from build123d import *

# Parameters (mm, degrees)
SKETCH4_W           = 30
SKETCH4_H           = 17.5
SKETCH4_R           = 2
BOSS_EXTRUDE2_DEPTH = 5
SKETCH5_W           = 30
SKETCH5_H           = 5
BOSS_EXTRUDE3_DEPTH = 15


with BuildPart() as part:
    # Sketch4 → Boss-Extrude2 (new body)
    with BuildSketch(Plane.XY):
        with Locations((0, 1.25)):
            Rectangle(SKETCH4_W, SKETCH4_H)
        with Locations((10.86, -3.5)):
            Circle(SKETCH4_R, mode=Mode.SUBTRACT)
        with Locations(Location((-10.86, -3.5, 0), (0, 0, 180))):
            Circle(SKETCH4_R, mode=Mode.SUBTRACT)
    extrude(amount=BOSS_EXTRUDE2_DEPTH)

    # Sketch5 → Boss-Extrude3 (add)
    with BuildSketch(Plane.XY):
        with Locations((0, 12.5)):
            Rectangle(SKETCH5_W, SKETCH5_H)
    extrude(amount=BOSS_EXTRUDE3_DEPTH)


solid = part.part
For this review, take the finished solid that the model builds, in its own axes (mm). A direction names the side the tool comes from. Give positions to 0.01 mm unless a question says otherwise; leave off trailing zeros. Order: outer loops, then holes, each group sorted by start corner. A loop starts at its lowest first (then second) coordinate and runs counter-clockwise, first axis right, second up. Notation, with made-up numbers: M 1,-17.5 L 55,-17.5 A13 cw 55,0.5 Z; hole C -0.5,59.5 d7. An arc over 180 degrees is marked long. Answer in a Markdown table with one row per item. Add a question column.
(1) Consider section C-C on z = 3.5. State the section outline as (x, y) points, and give its area (3 significant figures).
(2) Consider section A-A on y = -3.5. State the section outline as (x, z) points.
(3) Consider section B-B on x = 10.75. State the section outline as (y, z) points.
(4) Wall thickness on probe 1 along Y at (x, z) = (10.86, 3.7); probe 2 along Y at (x, z) = (13, 6.75); probe 3 along Z at (x, y) = (5.25, -5.5): over which ranges is each line inside the solid? List them lowest first. Write a range as [from, to].
(5) For faces 1 (the face through (0, 1, 5)), 2 (the face through (-8.862, -3.588, 2.465)), list the 3-axis set-ups (+Z, -Z, +X, -X, +Y, -Y) from which the entire face can be reached by the end or side of a thin tool; tool diameter is ignored.
(6) For pin 1 (9 mm diameter, centred on x = 7.5, y = 4, fed in from +Z), flat-tipped, find the tip position at first contact; note if it passes through.
(7) Mouldability with a two-part tool opening along X and no side actions: class faces 3 (the face through (8.862, -3.412, 2.465)), 4 (the face through (-15, 6, 4)), 5 (the face through (0, 10, 10)), 6 (the face through (15, 6, 4)) as +X half, -X half, draft (parallel to the pull), parting line (faces both ways), or undercut.
(8) Consider section D-D on x = 2.5. State the section outline as (y, z) points.
Evaluation:
| question | item | result |
|---|---|---|
| 1 | outline | M -15,-7.5 L 15,-7.5 L 15,15 L -15,15 Z; hole C -10.86,-3.5 d4; hole C 10.86,-3.5 d4 |
| 1 | area | 650 mm^2 |
| 2 | outline | M -15,0 L -12.86,0 L -12.86,5 L -15,5 Z; M -8.86,0 L 8.86,0 L 8.86,5 L -8.86,5 Z; M 12.86,0 L 15,0 L 15,5 L 12.86,5 Z |
| 3 | outline | M -7.5,0 L -5.5,0 L -5.5,5 L -7.5,5 Z; M -1.5,0 L 15,0 L 15,15 L 10,15 L 10,5 L -1.5,5 Z |
| 4 | probe 1 | y = [-7.5, -5.5], [-1.5, 15] |
| 4 | probe 2 | y = [10, 15] |
| 4 | probe 3 | z = [0, 5] |
| 5 | face 1 | +Z, +X, -X, -Y |
| 5 | face 2 | +Z, -Z |
| 6 | pin 1 | stops at z = 5 |
| 7 | face 3 | undercut |
| 7 | face 4 | -X half |
| 7 | face 5 | draft |
| 7 | face 6 | +X half |
| 8 | outline | M -7.5,0 L 15,0 L 15,15 L 10,15 L 10,5 L -7.5,5 Z |
